Could you check a few things on this model? Use its own coordinates, in mm. A direction names the side the tool comes from. Coordinates: 2 decimals unless noted, no trailing zeros. Order: outer loops, then holes, each group sorted by start corner. A loop starts at its lowest first (then second) coordinate and runs counter-clockwise, first axis right, second up. Notation, with made-up numbers: (79, 31.5) -> (124, 31.5) arc R37 cw to (124, 69.5) -> close; hole circle Ø7 at (-9.75, -8). An arc over 180 degrees is marked (long way). Put each result on its own line as item: value. Start each with the question number.
Q1. If we section it at D-D (x = -11.5): Please give me the cut outline in (y, z).
Q2. If we section it at C-C (y = 10): Please give me the cut outline in (x, z).
Q3. Will these pins go through, and if not, where does the flat tip stop? pin 1 (1 mm diameter, centred on x = 30.69, y = -3.81, fed in from +Z); pin 2 (2.5 mm diameter, centred on x = 18.5, y = 3.81, fed in from -Z); pin 3 (0.9 mm diameter, centred on x = 17.5, z = 2, fed in from +Y).
Q4. If we section it at A-A (y = 0): Please give me the cut outline in (x, z), and give its area (3 significant figures).
Q5. Please list where these lines run through material, in increasing order: line 1 along X through (y, z) = (0.25, 0.35); line 2 along X through (y, z) = (-2.25, 2.9); line 3 along Y through (x, z) = (26, 1.15).
Q6. If we section it at B-B (z = 1.5): Count the separate pieces of the cut face and the enclosed holes in it, and give its area (3 significant figures).
Q7. For faces 4 (the face through (13, 9, 1)), 5 (the face through (5, 2, 3)), 6 (the face through (-16.752, 11, 1)), which set-ups out of +Z, -Z, +X, -X, +Y, -Y let a thin tool reach every point of the face, with its end or its side?
Q8. We'd pull the mould along X, two halves only. Please class faces 1 (the face through (-3, 12, 1)), 2 (the face through (22.18, 7.04, 1.48)), 3 (the face through (33.596, 0.198, 1.479)): +X half, -X half, draft (parallel to the pull), parting line (faces both ways), or undercut.
from build123d import *

# Parameters (mm, degrees)
ESQUISSE1_R        = 4.5
ESQUISSE1_R_2      = 0.8
BOSS_EXTRU_1_DEPTH = 3


with BuildPart() as part:
    # Esquisse1 → Boss.-Extru.1 (new body)
    with BuildSketch(Plane.XY):
        with BuildLine():
            Line((1.597834667, 9), (24.597834667, 9))
            ThreePointArc((24.597834667, 9), (33.597834667, 0), (24.597834667, -9))
            Line((24.597834667, -9), (-25.402165333, -9))
            Line((-25.402165333, -9), (-25.402165333, 12))
            Line((-25.402165333, 12), (-16.752165333, 12))
            Line((-16.752165333, 12), (-16.752165333, 9))
            Line((-16.752165333, 9), (-7.052165333, 9))
            Line((-7.052165333, 9), (-7.052165333, 12))
            Line((-7.052165333, 12), (1.597834667, 12))
            Line((1.597834667, 12), (1.597834667, 9))
        make_face()
        with Locations((24.597834667, 0)):
            Circle(ESQUISSE1_R, mode=Mode.SUBTRACT)
        with Locations((22.97907079, 7)):
            Circle(ESQUISSE1_R_2, mode=Mode.SUBTRACT)
        with Locations((28.402943221, 6.094386383)):
            Circle(ESQUISSE1_R_2, mode=Mode.SUBTRACT)
        with Locations((31.597834667, 1.618763877)):
            Circle(ESQUISSE1_R_2, mode=Mode.SUBTRACT)
        with Locations((30.69222105, -3.805108554)):
            Circle(ESQUISSE1_R_2, mode=Mode.SUBTRACT)
        with Locations((26.216598544, -7)):
            Circle(ESQUISSE1_R_2, mode=Mode.SUBTRACT)
        with Locations((20.792726113, -6.094386383)):
            Circle(ESQUISSE1_R_2, mode=Mode.SUBTRACT)
        with Locations((17.597834667, -1.618763877)):
            Circle(ESQUISSE1_R_2, mode=Mode.SUBTRACT)
        with Locations((18.503448284, 3.805108554)):
            Circle(ESQUISSE1_R_2, mode=Mode.SUBTRACT)
    extrude(amount=BOSS_EXTRU_1_DEPTH)


solid = part.part
The answers:
1. outline: (-9, 0) -> (9, 0) -> (9, 3) -> (-9, 3) -> close
2. outline: (-25.4, 0) -> (-16.75, 0) -> (-16.75, 3) -> (-25.4, 3) -> close; (-7.05, 0) -> (1.6, 0) -> (1.6, 3) -> (-7.05, 3) -> close
3. pin 1: through
3. pin 2: z = 0
3. pin 3: y = 9
4. outline: (-25.4, 0) -> (20.1, 0) -> (20.1, 3) -> (-25.4, 3) -> close; (29.1, 0) -> (33.6, 0) -> (33.6, 3) -> (29.1, 3) -> close
4. area: 150 mm^2
5. line 1: -25.4 to 20.1, 29.09 to 33.59
5. line 2: -25.4 to 17.11, 18.09 to 20.7, 28.49 to 33.31
5. line 3: -8.89 to -7.77, -6.23 to -4.28, 4.28 to 8.89
6. separate pieces: 1
6. enclosed holes: 9
6. area: 999 mm^2
7. face 4: +Z, -Z, +X, +Y
7. face 5: +Z, +X, -X, +Y, -Y
7. face 6: +Z, -Z, +Y
8. face 1: draft
8. face 2: undercut
8. face 3: +X half
